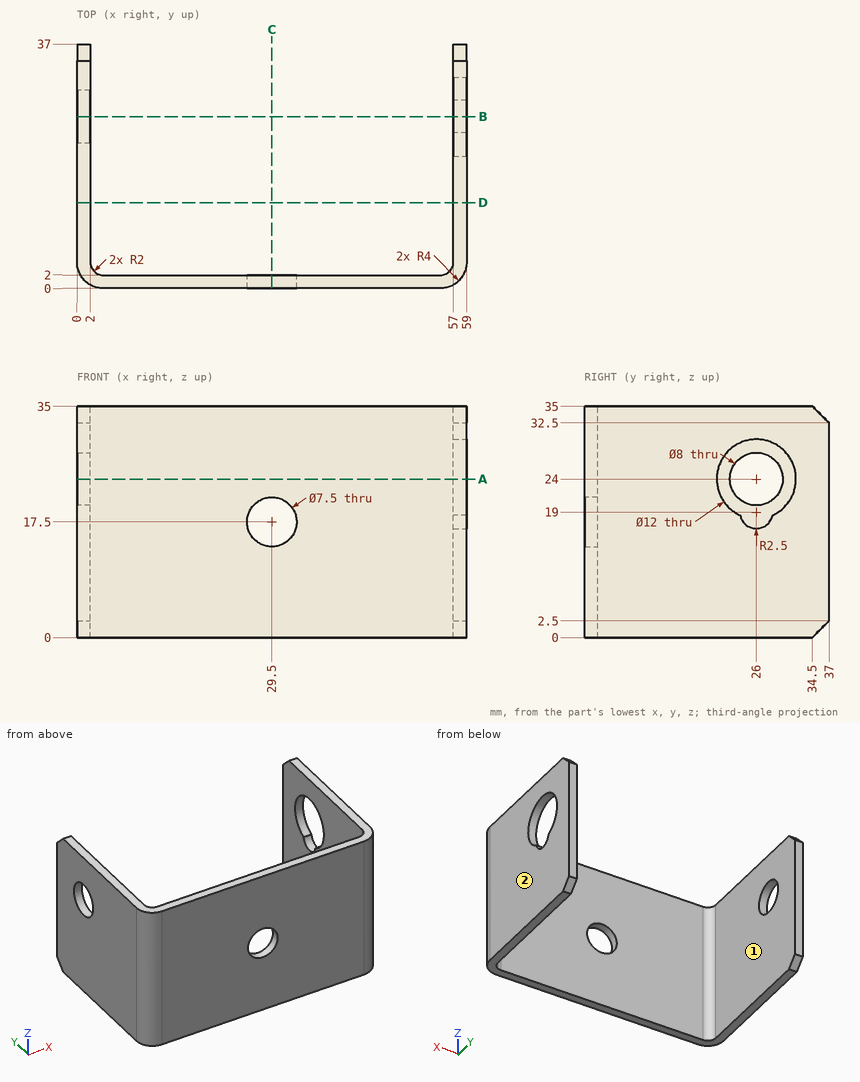
Here's the drawing with two shaded views (mm, measured from the low corner). I have some questions. A direction names the side the tool comes from. Give positions to 0.01 mm unless a question says otherwise; leave off trailing zeros. Write each loop counter-clockwise with the first axis right and the second up, starting at its lowest first coordinate (ties: lowest second). Pieces come first, ordered by that corner, then holes. Notation, with made-up numbers: (70.5, 72.5) -> (93.5, 72.5) arc R18 cw to (93.5, 83.5) -> close; hole circle Ø3 at (27, 4.25). An arc over 180 degrees is marked (long way). Answer as a JSON object with one key per item and string values. Group by question number.
Item 1: Suppose I cut it at C-C (x = 29.5). Please give me the cut outline in (y, z).
Item 2: Suppose I cut it at D-D (y = 13). Please give me the cut outline in (x, z), plus the area to 3 significant figures.
Item 3: Please list where these lines run through material, in increasing order: line 1 (Z direction, x = 57.6, y = 26); line 2 (X direction, y = 14.5, z = 24.5); line 3 (Y direction, x = 47, z = 6). Write a range as [from, to].
Item 4: For the marked faces 1 and 2, which set-ups out of +Z, -Z, +X, -X, +Y, -Y let a thin tool reach every point of the face, with its end or its side?
Item 5: Suppose I cut it at A-A (z = 24). Please give me the cut outline in (x, y), plus the area to 3 significant figures.
Item 6: Suppose I cut it at B-B (y = 26). Please give me the cut outline in (x, z).
Item 7: I'm going to push flat-ended pins straight in: P1, Ø13, axis at y = 26, z = 24, coming from the -X side; P2, Ø9.5, axis at y = 26, z = 24, coming from the +X side; P3, Ø4.5, axis at x = 29.5, z = 17.5, coming from the +Y side. Where does each tip first touch, or does it pass through?
Findings:
{
 "1": {"outline": "(0, 0) -> (2, 0) -> (2, 13.75) -> (0, 13.75) -> close; (0, 21.25) -> (2, 21.25) -> (2, 35) -> (0, 35) -> close"},
 "2": {"outline": "(0, 0) -> (2, 0) -> (2, 35) -> (0, 35) -> close; (57, 0) -> (59, 0) -> (59, 35) -> (57, 35) -> close", "area": "140 mm²"},
 "3": {"line 1": "z = [0, 16.5], [30, 35]", "line 2": "x = [0, 2], [57, 59]", "line 3": "y = [0, 2]"},
 "4": {"face 1": "+Z, -Z, +Y", "face 2": "+Z, -Z, +X, +Y, -Y"},
 "5": {"outline": "(0, 4) arc R4 ccw to (4, 0) -> (55, 0) arc R4 ccw to (59, 4) -> (59, 20) -> (57, 20) -> (57, 4) arc R2 cw to (55, 2) -> (4, 2) arc R2 cw to (2, 4) -> (2, 22) -> (0, 22) -> close; (0, 30) -> (2, 30) -> (2, 37) -> (0, 37) -> close; (57, 32) -> (59, 32) -> (59, 37) -> (57, 37) -> close", "area": "213 mm²"},
 "6": {"outline": "(0, 0) -> (2, 0) -> (2, 20) -> (0, 20) -> close; (0, 28) -> (2, 28) -> (2, 35) -> (0, 35) -> close; (57, 0) -> (59, 0) -> (59, 16.5) -> (57, 16.5) -> close; (57, 30) -> (59, 30) -> (59, 35) -> (57, 35) -> close"},
 "7": {"P1": "stops at x = 0", "P2": "stops at x = 2", "P3": "passes through"}
}
